```python
from build123d import *


with BuildPart() as part:
    # Sketch → Revolution (revolve)
    with BuildSketch(Plane.XZ):
        with BuildLine():
            Line((0, 0), (0.75, 0))
            Line((0.75, 0), (1.350002, 0.8))
            Line((1.350002, 0.8), (3.1, 0.8))
            Line((3.1, 0.8), (3.1, 1.2))
            Line((2.6, 1.2), (3.1, 1.2))
            Line((2.6, 2.15), (2.6, 1.2))
            ThreePointArc((2.6, 2.15), (2.38033, 2.68033), (1.85, 2.9))
            Line((1.85, 2.9), (0, 2.9))
            Line((0, 2.9), (0, 0))
        make_face()
    revolve(axis=Axis((0, 0, 0), (0, 0, 1)))


solid = part.part
```
Input: part model. Units: mm. Frame: model coordinates. A direction names the side the tool comes from. Coordinates: 2 decimals unless noted, no trailing zeros. Write each loop counter-clockwise with the first axis right and the second up, starting at its lowest first coordinate (ties: lowest second). Pieces come first, ordered by that corner, then holes. Notation, with made-up numbers: (80, 55.25) -> (95, 55.25) arc R30 ccw to (95, 93.25) -> close; hole circle Ø7 at (-29.5, 41). An arc over 180 degrees is marked (long way). Answer as a JSON object with one key per item and string values.
1. Access query for faces 1 (the face through (-1.33, 0.73, 0.8)), 2 (the face through (-0.338, 2.578, 1.668)), 3 (the face through (1.43, -2.75, 1)). Directions: +Z, -Z, +X, -X, +Y, -Y. A direction counts if a zero-diameter tool reaches every point of the face in a straight line with its end or side. Return the directions, or none.
Result set:
{"face 1": "-Z", "face 2": "+Z", "face 3": "+Z, -Z"}
2. Section B-B on z = 1.05. Return the cut outline in (x, y), then the cut area to 3 significant figures.
Result set:
{"outline": "circle Ø6.2 at (0, 0)", "area": "30.2 mm2"}
3. Section D-D on z = 0.2. Return the cut outline in (x, y).
Result set:
{"outline": "circle Ø1.8 at (0, 0)"}
4. First-contact query: P1, Ø1.5, axis at x = 1.5, y = -0.5, coming from the -Z side; P2, Ø1.5, axis at x = -1.5, y = -2.5, coming from the +Z side; P3, Ø1, axis at x = 2.5, z = 1.5, coming from the +Y side. Flat tips, straight axial feed; report the tip coordinate or a pass-through.
Result set:
{"P1": "stops at z = 0.11", "P2": "stops at z = 2.83", "P3": "stops at y = 2.28"}
5. Material intervals for line 1 (Z direction, x = -1.5, y = -0.75); line 2 (Z direction, x = 2, y = 2); line 3 (Y direction, x = 0.25, z = 1.35), sorted ascending. Write a range as from..to.
Result set:
{"line 1": "z = 0.8..2.9", "line 2": "z = 0.8..1.2", "line 3": "y = -2.59..2.59"}
6. Section C-C on y = 2.75. Return the cut outline in (x, z), then the cut area to 3 significant figures.
Result set:
{"outline": "(-1.43, 0.8) -> (1.43, 0.8) -> (1.43, 1.2) -> (-1.43, 1.2) -> close", "area": "1.14 mm2"}
7. Section A-A on x = 0. Return the cut outline in (y, z).
Result set:
{"outline": "(-3.1, 0.8) -> (-1.35, 0.8) -> (-0.75, 0) -> (0.75, 0) -> (1.35, 0.8) -> (3.1, 0.8) -> (3.1, 1.2) -> (2.6, 1.2) -> (2.6, 2.15) arc R0.75 ccw to (1.85, 2.9) -> (-1.85, 2.9) arc R0.75 ccw to (-2.6, 2.15) -> (-2.6, 1.2) -> (-3.1, 1.2) -> close"}
